from build123d import *

# Parameters (mm, degrees)
BOSS_EXTRUDE1_DEPTH = 5
SKETCH2_R           = 1.5
CUT_EXTRUDE1_DEPTH  = 41.708230126
SKETCH3_W           = 5
SKETCH3_H           = 5
BOSS_EXTRUDE2_DEPTH = 47
BOSS_EXTRUDE3_DEPTH = 5
SKETCH5_R           = 1.5
CUT_EXTRUDE2_DEPTH  = 77.27686412
BOSS_EXTRUDE4_DEPTH = 12.5
SKETCH10_W          = 5
SKETCH10_H          = 5
BOSS_EXTRUDE5_DEPTH = 14.6
BOSS_EXTRUDE6_DEPTH = 5


with BuildPart() as part:
    # Sketch1 → Boss-Extrude1 (new body)
    with BuildSketch(Plane.XY):
        Polygon((0, 0), (0, 25), (-3.65, 25), (-3.65, 39.6), (1.35, 39.6), (1.35, 30), (5, 30), (5, -5), (-8, -5), (-8, 0), align=None)
    extrude(amount=BOSS_EXTRUDE1_DEPTH)

    # Sketch2 → Cut-Extrude1 (cut, through all)
    with BuildSketch(Plane(origin=(0, 0, 0), x_dir=(1, 0, 0), z_dir=(0, 1, 0))):
        with Locations(Location((-4, -2.5, 0), (0, 0, 270))):
            Circle(SKETCH2_R)
    extrude(amount=-CUT_EXTRUDE1_DEPTH, mode=Mode.SUBTRACT)

    # Sketch3 → Boss-Extrude2 (add)
    with BuildSketch(Plane(origin=(5, 0, 0), x_dir=(0, 0, -1), z_dir=(1, 0, 0))):
        with Locations((-2.5, 27.5)):
            Rectangle(SKETCH3_W, SKETCH3_H)
    extrude(amount=BOSS_EXTRUDE2_DEPTH)

    # Sketch4 → Boss-Extrude3 (add)
    with BuildSketch(Plane(origin=(0, 0, 0), x_dir=(-1, 0, 0), z_dir=(0, 0, -1))):
        Polygon((-52, 30), (-55.65, 30), (-55.65, 39.379320009), (-60.65, 39.379320009), (-60.65, 25), (-57, 25), (-57, 0), (-65, 0), (-65, -4.395887534), (-52, -4.395887534), (-52, 25), align=None)
    extrude(amount=-BOSS_EXTRUDE3_DEPTH)

    # Sketch5 → Cut-Extrude2 (cut, through all)
    with BuildSketch(Plane(origin=(0, 0, 0), x_dir=(1, 0, 0), z_dir=(0, 1, 0))):
        with Locations(Location((61, -2.5, 0), (0, 0, 180))):
            Circle(SKETCH5_R)
    extrude(amount=-CUT_EXTRUDE2_DEPTH, mode=Mode.SUBTRACT)

    # Sketch7 → Boss-Extrude4 (add)
    with BuildSketch(Plane.XY.offset(5)):
        Polygon((28.5, 30), (31, 30), (31, 25), (26, 25), (26, 30), align=None)
    extrude(amount=BOSS_EXTRUDE4_DEPTH)

    # Sketch10 → Boss-Extrude5 (add)
    with BuildSketch(Plane(origin=(0, 25, 0), x_dir=(-1, 0, 0), z_dir=(0, -1, 0))):
        with Locations((-28.5, -20)):
            Rectangle(SKETCH10_W, SKETCH10_H)
    extrude(amount=-BOSS_EXTRUDE5_DEPTH)

    # Sketch11 → Boss-Extrude6 (add)
    with BuildSketch(Plane(origin=(0, 39.6, 0), x_dir=(1, 0, 0), z_dir=(0, 1, 0))):
        Polygon((26, -17.5), (26, -14.5), (31, -14.5), (31, -22.5), (26, -22.5), align=None)
    extrude(amount=BOSS_EXTRUDE6_DEPTH)


solid = part.part
Verification items for the finished model (mm, model axes). A direction names the side the tool comes from. Round coordinates to 2 decimals unless told otherwise and drop trailing zeros. Write each loop counter-clockwise with the first axis right and the second up, starting at its lowest first coordinate (ties: lowest second). Pieces come first, ordered by that corner, then holes.
(1) Depth check by flat-ended pin: pin 1 Ø4 at (x, z) = (60, 3) entering from +Y; pin 2 Ø5.5 at (x, z) = (-0.5, 1.5) entering from +Y; pin 3 Ø1.8 at (x, z) = (59, 2.5) entering from -Y; pin 4 Ø1.5 at (y, z) = (32, 15) entering from -X. Enter the tip coordinate at first touch or a pass-through.
Returned:
pin 1: stops at y = 39.38
pin 2: stops at y = 39.6
pin 3: stops at y = -4.4
pin 4: passes through
(2) Section check C-C (y = 34). Enter the section's corners in (x, z), plus the area to 3 significant figures.
Returned:
outline: (-3.65, 0) - (1.35, 0) - (1.35, 5) - (-3.65, 5) - close; (26, 17.5) - (31, 17.5) - (31, 22.5) - (26, 22.5) - close; (55.65, 0) - (60.65, 0) - (60.65, 5) - (55.65, 5) - close
area: 75.0 mm2
(3) Material ranges on line 1 (X direction, y = 36.5, z = 1.75); line 2 (Z direction, x = 61, y = -3.2); line 3 (X direction, y = 40, z = 20), recorded low to high.
Returned:
line 1: x = -3.65 to 1.35, 55.65 to 60.65
line 2: z = 0 to 1, 4 to 5
line 3: x = 26 to 31
(4) Section check A-A (z = 2.5). Enter the section's corners in (x, y).
Returned:
outline: (-8, -5) - (-5.5, -5) - (-5.5, 0) - (-8, 0) - close; (-3.65, 25) - (0, 25) - (0, 0) - (-2.5, 0) - (-2.5, -5) - (5, -5) - (5, 25) - (52, 25) - (52, -4.4) - (59.5, -4.4) - (59.5, 0) - (57, 0) - (57, 25) - (60.65, 25) - (60.65, 39.38) - (55.65, 39.38) - (55.65, 30) - (1.35, 30) - (1.35, 39.6) - (-3.65, 39.6) - close; (62.5, -4.4) - (65, -4.4) - (65, 0) - (62.5, 0) - close
(5) Mould release check, pull along Y, two halves, no side actions. Record for faces 4 (the flat face through (29, 39.6, 16)), 5 (the flat face through (5, 10, 2)), 6 (the flat face through (58, 39.379, 2)): pulls with the +Y half, pulls with the -Y half, needs draft (parallel to the pull), parting line crosses it, or undercut.
Returned:
face 4: undercut
face 5: needs draft
face 6: pulls with the +Y half
(6) Section check D-D (y = -1). Enter the section's corners in (x, z), plus the area to 3 significant figures.
Returned:
outline: (-8, 0) - (5, 0) - (5, 5) - (-8, 5) - close; (52, 0) - (65, 0) - (65, 5) - (52, 5) - close; hole circle Ø3 at (-4, 2.5); hole circle Ø3 at (61, 2.5)
area: 116 mm2
(7) Access from +Z, -Z, +X, -X, +Y, -Y to the whole of each face (thin tool, end or side, straight path). Record for faces 1 (the cylindrical face through (59.57, -2.17, 2.95)), 2 (the flat face through (59, 25, 2)), 3 (the flat face through (1.35, 35, 2)).
Returned:
face 1: -Y
face 2: +Z, -Z, +X
face 3: +Z, -Z, +Y
(8) Section check B-B (y = 22). Enter the section's corners in (x, z), plus the area to 3 significant figures.
Returned:
outline: (0, 0) - (5, 0) - (5, 5) - (0, 5) - close; (52, 0) - (57, 0) - (57, 5) - (52, 5) - close
area: 50.0 mm2
